The listing builds one solid part. Answer for the finished solid, in the listing's coordinates (mm). Coordinates: 2 decimals unless noted, no trailing zeros. Order: outer loops, then holes, each group sorted by start corner. A loop starts at its lowest first (then second) coordinate and runs counter-clockwise, first axis right, second up.
from build123d import *

# Parameters (mm, degrees)
F1_R     = 6.35
F1_R_2   = 11.0998
F2_DEPTH = 12.7


with BuildPart() as f2:
    # F1 (on face) → F2 (new body)
    with BuildSketch(Plane.XY):
        with BuildLine():
            ThreePointArc((33.339887, 52.153976), (0, 61.8998), (-33.339887, 52.153976))
            ThreePointArc((-33.339887, 52.153976), (-31.01255, 23.579573), (-59.169025, 18.18273))
            ThreePointArc((-59.169025, 18.18273), (-61.899657, 0.132973), (-59.246599, -17.92835))
            ThreePointArc((-59.246599, -17.92835), (-29.299818, -22.178176), (-33.339887, -52.153976))
            ThreePointArc((-33.339887, -52.153976), (0, -61.8998), (33.339887, -52.153976))
            ThreePointArc((33.339887, -52.153976), (29.299818, -22.178176), (59.246599, -17.92835))
            ThreePointArc((59.246599, -17.92835), (61.899657, 0.132973), (59.169025, 18.18273))
            ThreePointArc((59.169025, 18.18273), (31.01255, 23.579573), (33.339887, 52.153976))
        make_face()
        with Locations((-46.4058, 0)):
            Circle(F1_R, mode=Mode.SUBTRACT)
        with Locations((0, -46.4058)):
            Circle(F1_R, mode=Mode.SUBTRACT)
        Circle(F1_R_2, mode=Mode.SUBTRACT)
        with Locations((46.4058, 0)):
            Circle(F1_R, mode=Mode.SUBTRACT)
        with Locations((0, 46.4058)):
            Circle(F1_R, mode=Mode.SUBTRACT)
    extrude(amount=F2_DEPTH)


solid = f2.part
1) Section D-D (z = 5.5) is taken. Give the vertices of the cut face in (x, y).
2) Section A-A (y = 0) is taken. Give the vertices of the cut face in (x, z).
3) Consider L1, parallel to X at y = -3, z = 7.75; L2, parallel to Y at x = 52, z = 10.75; L3, parallel to Y at x = -2, z = 3. Determine where each line is inside the solid, lowest interval first.
4) Each of these flat-tipped pins is pushed along its axis until it touches: P1, Ø1, axis at y = 21, z = 6.5, coming from the -X side; P2, Ø4, axis at x = -23.5, y = -43.5, coming from the -Z side; P3, Ø4, axis at y = 37, z = 6, coming from the +X side; P4, Ø1.5, axis at y = 15, z = 7, coming from the +X side. Where does it stop, or does it pass through?
5) Determine the mould class of faces 1 (the face through (61.9, -0.1, 6.3)), 2 (the face through (31.282, 23.232, 6.261)), 3 (the face through (13, 1, 12.7)) for opening direction X: released by +X, released by -X, zero draft, split by the parting line, or undercut.
6) Section C-C (x = -29.5) is taken. Give the vertices of the cut face in (y, z).
Filled sheet:
1. outline: (-59.25, -17.93) arc R21.46 cw to (-33.34, -52.15) arc R61.9 ccw to (33.34, -52.15) arc R21.46 cw to (59.25, -17.93) arc R61.9 ccw to (59.17, 18.18) arc R21.46 cw to (33.34, 52.15) arc R61.9 ccw to (-33.34, 52.15) arc R21.46 cw to (-59.17, 18.18) arc R61.9 ccw to start; hole circle Ø12.7 at (-46.41, 0); hole circle Ø22.2 at (0, 0); hole circle Ø12.7 at (0, -46.41); hole circle Ø12.7 at (0, 46.41); hole circle Ø12.7 at (46.41, 0)
2. outline: (-61.9, 0) - (-52.76, 0) - (-52.76, 12.7) - (-61.9, 12.7) - close; (-40.06, 0) - (-11.1, 0) - (-11.1, 12.7) - (-40.06, 12.7) - close; (11.1, 0) - (40.06, 0) - (40.06, 12.7) - (11.1, 12.7) - close; (52.76, 0) - (61.9, 0) - (61.9, 12.7) - (52.76, 12.7) - close
3. L1: x = -61.83 to -52, -40.81 to -10.69, 10.69 to 40.81, 52 to 61.83
3. L2: y = -14.41 to -3, 3 to 15.46
3. L3: y = -61.87 to -52.43, -40.38 to -10.92, 10.92 to 40.38, 52.43 to 61.87
4. P1: stops at x = -33.87
4. P2: stops at z = 0
4. P3: stops at x = 26.77
4. P4: stops at x = 60.24
5. face 1: released by +X
5. face 2: undercut
5. face 3: zero draft
6. outline: (-54.42, 0) - (-48.35, 0) - (-48.35, 12.7) - (-54.42, 12.7) - close; (-21.92, 0) - (25.86, 0) - (25.86, 12.7) - (-21.92, 12.7) - close; (47.28, 0) - (54.42, 0) - (54.42, 12.7) - (47.28, 12.7) - close
